Part model, mm, in its own coordinate system. Face numbers are marked on the shaded views. A direction names the side the tool comes from. Round coordinates to 2 decimals unless told otherwise and drop trailing zeros. Loops run counter-clockwise (first coordinate to the right, second up) from the corner with the lowest first, then second, coordinate; pieces in that order, holes last. Notation, with made-up numbers: (58.25, 52) -> (73.25, 52) arc R14 ccw to (73.25, 75) -> close; hole circle Ø3 at (24, -12.5). An arc over 180 degrees is marked (long way). Use a Markdown table: item, result. Add a question column.
Item 1: Cut at C-C, the plane y = 51.5. List the corners of the cut face in (x, z), plus the area to 3 significant figures.
Item 2: Probe line 1 (X direction, y = 4, z = 0); line 2 (X direction, y = 50, z = 0); line 3 (Y direction, x = 27.5, z = 9). List the from-to ranges inside material, lowest first. Write a range as [from, to].
Item 3: Flat gauge pins, fed straight in: pin 1 (15.5 mm diameter, centred on x = 0, z = 0, fed in from -Y); pin 2 (3 mm diameter, centred on x = 15.5, y = 60.5, fed in from -Z); pin 3 (12 mm diameter, centred on y = 8.5, z = 26, fed in from -X); pin 4 (1.5 mm diameter, centred on x = 26.5, z = 1, fed in from +Y). Where does each tip first touch, or does it go through?
Item 4: Which spindle directions (+Z, -Z, +X, -X, +Y, -Y) get a long thin tool onto all of the face, cutting with end or side? Do the marked faces 4 and 5. Say none if no direction does.
Item 5: Two-plate mould, pull along Z, no slides. Class the marked faces 1, 2 and 3: pulls with the +Z half, pulls with the -Z half, needs draft (parallel to the pull), parting line crosses it, or undercut.
Item 6: Cut at D-D, the plane x = -9. List the corners of the cut face in (y, z), plus the area to 3 significant figures.
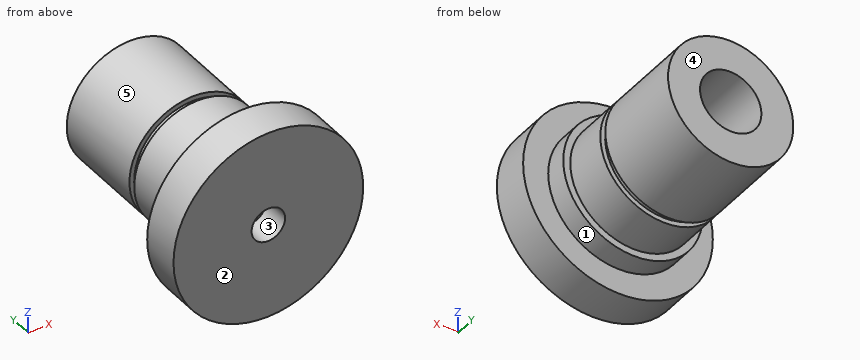
```python
from build123d import *


with BuildPart() as part:
    # Sketch1 → Revolve1 (revolve)
    with BuildSketch(Plane.XY, mode=Mode.PRIVATE) as revolve1_sk:
        Polygon((-6, 0), (-34, 0), (-34, 14), (-25, 14), (-25, 74), (-11, 74), (-11, 30), (-3.25, 30), (-3.25, 10), (-6, 10), align=None)
    revolve(revolve1_sk.sketch.rotate(Axis((0, 0, 0), (0, 1, 0)), 270), axis=Axis((0, 0, 0), (0, 1, 0)))

    # Sketch3 → Cut-Revolve1 (revolve, cut)
    with BuildSketch(Plane.XY, mode=Mode.PRIVATE) as cut_revolve1_sk:
        Polygon((22.45, 74), (22.45, 40.6), (20.75, 40.6), (20.75, 38), (22.5, 38), (22.5, 22), (25, 22), (25, 74), align=None)
    revolve(cut_revolve1_sk.sketch.rotate(Axis((0, 0, 0), (0, 1, 0)), 90), axis=Axis((0, 0, 0), (0, 1, 0)), mode=Mode.SUBTRACT)


solid = part.part
```
A:
| question | item | result |
|---|---|---|
| 1 | outline | circle Ø44.9 at (0, 0); hole circle Ø22 at (0, 0) |
| 1 | area | 1,200 mm^2 |
| 2 | line 1 | x = [-34, -6], [6, 34] |
| 2 | line 2 | x = [-22.45, -11], [11, 22.45] |
| 2 | line 3 | y = [0, 14] |
| 3 | pin 1 | stops at y = 0 |
| 3 | pin 2 | stops at z = -17.55 |
| 3 | pin 3 | stops at x = -27.5 |
| 3 | pin 4 | stops at y = 14 |
| 4 | face 4 | +Z, -Z, +X, -X, +Y |
| 4 | face 5 | +Y |
| 5 | face 1 | parting line crosses it |
| 5 | face 2 | needs draft |
| 5 | face 3 | undercut |
| 6 | outline | (0, -32.79) -> (14, -32.79) -> (14, -23.32) -> (22, -23.32) -> (22, -20.62) -> (38, -20.62) -> (38, -18.7) -> (40.6, -18.7) -> (40.6, -20.57) -> (74, -20.57) -> (74, -6.32) -> (30, -6.32) -> (30, 6.32) -> (74, 6.32) -> (74, 20.57) -> (40.6, 20.57) -> (40.6, 18.7) -> (38, 18.7) -> (38, 20.62) -> (22, 20.62) -> (22, 23.32) -> (14, 23.32) -> (14, 32.79) -> (0, 32.79) -> close |
| 6 | area | 2,870 mm^2 |
